from build123d import *

# Parameters (mm, degrees)
SKETCH1_W                    = 19.8
SKETCH1_H                    = 10.6
BOSS_EXTRUDE1_DEPTH          = 6.4
SKETCH2_W                    = 10.8
SKETCH2_H                    = 0.7
CUT_EXTRUDE1_DEPTH           = 18.703389506
SKETCH3_W                    = 3.3
SKETCH3_H                    = 0.4
CUT_EXTRUDE2_DEPTH           = 18.703389506
SKETCH4_W                    = 5.9
SKETCH4_H                    = 0.4
CUT_EXTRUDE3_DEPTH           = 18.703389506
SKETCH5_W                    = 3.4
SKETCH5_H                    = 0.4
CUT_EXTRUDE4_DEPTH           = 18.703389506
CUT_EXTRUDE5_DEPTH           = 18.703389506
BOSS_EXTRUDE2_DEPTH          = 3.2
SKETCH8_W                    = 0.5
SKETCH8_H                    = 3.2
BOSS_EXTRUDE3_DEPTH          = 3.9
SKETCH9_W                    = 0.5
SKETCH9_H                    = 3.2
BOSS_EXTRUDE4_DEPTH          = 3.9
SKETCH10_W                   = 0.5
SKETCH10_H                   = 3.2
BOSS_EXTRUDE5_DEPTH          = 3.9
DRAFT1_ANGLE                 = 45
DRAFT2_ANGLE                 = 45
DRAFT3_ANGLE                 = 45
DRAFT4_ANGLE                 = 45
F_2_35_2_35_DIAMETER_HOLE1_D = 2.35


with BuildPart() as part:
    # Sketch1 → Boss-Extrude1 (new body)
    with BuildSketch(Plane.XY.offset(3.2)):
        with Locations((-4.7, 2.4)):
            Rectangle(SKETCH1_W, SKETCH1_H)
    extrude(amount=-BOSS_EXTRUDE1_DEPTH)

    # Sketch2 → Cut-Extrude1 (cut, through all)
    with BuildSketch(Plane(origin=(0, 0, -3.2), x_dir=(-1, 0, 0), z_dir=(0, 0, -1))):
        with Locations((0.2, 7.35)):
            Rectangle(SKETCH2_W, SKETCH2_H)
    extrude(amount=-CUT_EXTRUDE1_DEPTH, mode=Mode.SUBTRACT)

    # Sketch3 → Cut-Extrude2 (cut, through all)
    with BuildSketch(Plane(origin=(0, 0, -3.2), x_dir=(-1, 0, 0), z_dir=(0, 0, -1))):
        with Locations((12.95, -2.7)):
            Rectangle(SKETCH3_W, SKETCH3_H)
    extrude(amount=-CUT_EXTRUDE2_DEPTH, mode=Mode.SUBTRACT)

    # Sketch4 → Cut-Extrude3 (cut, through all)
    with BuildSketch(Plane(origin=(0, 0, -3.2), x_dir=(-1, 0, 0), z_dir=(0, 0, -1))):
        with Locations((4.75, -2.7)):
            Rectangle(SKETCH4_W, SKETCH4_H)
    extrude(amount=-CUT_EXTRUDE3_DEPTH, mode=Mode.SUBTRACT)

    # Sketch5 → Cut-Extrude4 (cut, through all)
    with BuildSketch(Plane(origin=(0, 0, -3.2), x_dir=(-1, 0, 0), z_dir=(0, 0, -1))):
        with Locations((-3.5, -2.7)):
            Rectangle(SKETCH5_W, SKETCH5_H)
    extrude(amount=-CUT_EXTRUDE4_DEPTH, mode=Mode.SUBTRACT)

    # Sketch6 → Cut-Extrude5 (cut, through all)
    with BuildSketch(Plane(origin=(0, 0, -3.2), x_dir=(-1, 0, 0), z_dir=(0, 0, -1))):
        with BuildLine():
            Line((9.073531947, -1.175), (9.926468053, -1.175))
            ThreePointArc((9.926468053, -1.175), (10.75, 0), (9.926468053, 1.175))
            Line((9.926468053, 1.175), (9.073531947, 1.175))
            ThreePointArc((9.073531947, 1.175), (8.25, 0), (9.073531947, -1.175))
        make_face()
    extrude(amount=-CUT_EXTRUDE5_DEPTH, mode=Mode.SUBTRACT)

    # Sketch7 → Boss-Extrude2 (add)
    with BuildSketch(Plane.XY.offset(1.6)):
        with BuildLine():
            Line((-8.5, 7.825612234), (-8.5, 7.7))
            Line((-8.5, 7.7), (-6.5, 7.7))
            Line((-6.5, 7.7), (-6.5, 7.825612234))
            ThreePointArc((-6.5, 7.825612234), (-7.5, 8.362287276), (-8.5, 7.825612234))
        make_face()
    extrude(amount=-BOSS_EXTRUDE2_DEPTH)

    # Sketch8 → Boss-Extrude3 (add)
    with BuildSketch(Plane.XZ.offset(2.5)):
        with Locations((-3.95, 0)):
            Rectangle(SKETCH8_W, SKETCH8_H)
    extrude(amount=BOSS_EXTRUDE3_DEPTH)

    # Sketch9 → Boss-Extrude4 (add)
    with BuildSketch(Plane.XZ.offset(2.5)):
        with Locations((3.35, 0)):
            Rectangle(SKETCH9_W, SKETCH9_H)
    extrude(amount=BOSS_EXTRUDE4_DEPTH)

    # Sketch10 → Boss-Extrude5 (add)
    with BuildSketch(Plane.XZ.offset(2.5)):
        with Locations((-12.75, 0)):
            Rectangle(SKETCH10_W, SKETCH10_H)
    extrude(amount=BOSS_EXTRUDE5_DEPTH)

    # Draft1
    draft1_faces = [part.faces().sort_by_distance(p)[0] for p in [
        (-5.6, 7.35, 0),
    ]]
    draft(draft1_faces, Plane(origin=(5.2, 7.7, -3.2), x_dir=(1, 0, 0), z_dir=(0, 1, 0)), DRAFT1_ANGLE)

    # Draft2
    draft2_faces = [part.faces().sort_by_distance(p)[0] for p in [
        (1.8, -2.7, 0),
    ]]
    draft(draft2_faces, Plane(origin=(1.8, -2.5, 3.2), x_dir=(0, 0, -1), z_dir=(0, -1, 0)), DRAFT2_ANGLE)

    # Draft3
    draft3_faces = [part.faces().sort_by_distance(p)[0] for p in [
        (-11.3, -2.7, 0),
    ]]
    draft(draft3_faces, Plane(origin=(-14.6, -2.5, 3.2), x_dir=(0, 0, -1), z_dir=(0, -1, 0)), DRAFT3_ANGLE)

    # Draft4
    draft4_faces = [part.faces().sort_by_distance(p)[0] for p in [
        (-7.7, -2.7, 0),
        (-1.8, -2.7, 0),
    ]]
    draft(draft4_faces, Plane(origin=(-7.7, -2.5, 3.2), x_dir=(0, 0, -1), z_dir=(0, -1, 0)), DRAFT4_ANGLE)

    # Ø2.35 (2.35) Diameter Hole1 (through all)
    with Locations(Plane.XY.offset(3.2)):
        with Locations((0, 0)):
            Hole(F_2_35_2_35_DIAMETER_HOLE1_D / 2)


solid = part.part
The model under review builds one solid part; all positions refer to its coordinate system, in mm. A direction names the side the tool comes from. Give positions to 0.01 mm unless a question says otherwise; leave off trailing zeros. Loops run counter-clockwise (first coordinate to the right, second up) from the corner with the lowest first, then second, coordinate; pieces in that order, holes last. Notation, with made-up numbers: (-25.75, 41) -> (26.25, 41) arc R10 cw to (26.25, 46) -> close; hole circle Ø10 at (0.25, 15.25). An arc over 180 degrees is marked (long way). Answer as a JSON object with one key per item and string values. Group by question number.
Q1. Take a section at B-B (x = 0). Write out the cut boundary in (y, z) (3 decimals), plus the area to 3 significant figures.
Q2. Wall thickness on line 1 along X through (y, z) = (-4.25, -0.75); line 2 along X through (y, z) = (-2.75, 0.5); line 3 along Y through (x, z) = (0, -0.5) (3 decimals): over which ranges is each line inside the solid? List them lowest first.
Q3. Take a section at C-C (y = -4.5). Write out the cut boundary in (x, z).
Q4. Take a section at A-A (y = 0). Write out the cut boundary in (x, z) (3 decimals).
Q5. Draft analysis for pull direction Y (two halves, no side actions). For faces 6 (the flat face through (0, -2.9, 0)), 7 (the flat face through (-4.2, -4, 0)), 8 (the flat face through (0, 7, 0)), 9 (the cylindrical face through (0.25, -1.15, -0.04)), state which applies: pulls with the +Y half, pulls with the -Y half, needs draft (parallel to the pull), parting line crosses it, or undercut.
Q6. Insertion check: pin 1 (0.5 mm diameter, centred on x = -8, y = 8, fed in from -Z); pin 2 (2.5 mm diameter, centred on y = -5, z = 1, fed in from +X); pin 3 (1.5 mm diameter, centred on x = 1, z = 0, fed in from -Y). Each pin has a flat end and moves straight along its axis. Give the tip position at first contact, or say it passes through.
Q7. Take a section at D-D (z = -0.75). State how many separate pieces and enclosed holes the cut face has, plus the area to 3 significant figures.
Q8. Tool access review of faces 1 (the flat face through (-5, 2, 3.2)), 2 (the flat face through (-13, -4, 0)), 3 (the cylindrical face through (-10.75, -0.02, -0.04)), 4 (the flat face through (5.2, 2, 0)), 5 (the flat face through (3.1, -4, 0)): name each direction out of +Z, -Z, +X, -X, +Y, -Y from which nothing blocks a thin tool from reaching the whole face with its end or side.
Answer below:
{
 "1": {"outline": "(-2.9, -3.2) -> (-1.175, -3.2) -> (-1.175, 3.2) -> (-2.9, 3.2) -> close; (1.175, -3.2) -> (7, -3.2) -> (7, 3.2) -> (1.175, 3.2) -> close", "area": "48.3 mm2"},
 "2": {"line 1": "x = -13 to -12.5, -4.2 to -3.7, 3.1 to 3.6", "line 2": "x = -13 to -12.5, -11.05 to -7.95, -4.2 to -3.7, -1.55 to 1.55, 3.1 to 3.6", "line 3": "y = -2.9 to -1.175, 1.175 to 7"},
 "3": {"outline": "(-13, -1.6) -> (-12.5, -1.6) -> (-12.5, 1.6) -> (-13, 1.6) -> close; (-4.2, -1.6) -> (-3.7, -1.6) -> (-3.7, 1.6) -> (-4.2, 1.6) -> close; (3.1, -1.6) -> (3.6, -1.6) -> (3.6, 1.6) -> (3.1, 1.6) -> close"},
 "4": {"outline": "(-14.6, -3.2) -> (-10.75, -3.2) -> (-10.75, 3.2) -> (-14.6, 3.2) -> close; (-8.25, -3.2) -> (-1.175, -3.2) -> (-1.175, 3.2) -> (-8.25, 3.2) -> close; (1.175, -3.2) -> (5.2, -3.2) -> (5.2, 3.2) -> (1.175, 3.2) -> close"},
 "5": {"face 6": "pulls with the -Y half", "face 7": "needs draft", "face 8": "pulls with the +Y half", "face 9": "undercut"},
 "6": {"pin 1": "stops at z = -1.6", "pin 2": "stops at x = 3.6", "pin 3": "stops at y = -2.9"},
 "7": {"separate pieces": "1", "enclosed holes": "2", "area": "195 mm2"},
 "8": {"face 1": "+Z, +X, -X, +Y, -Y", "face 2": "+Z, -Z, -X, -Y", "face 3": "+Z, -Z", "face 4": "+Z, -Z, +X, +Y, -Y", "face 5": "+Z, -Z, -Y"}
}
